CAD build for the part. Positions are in the model's coordinates, mm. Face numbers are marked on the shaded views. Give positions to 0.01 mm unless a question says otherwise; leave off trailing zeros. Loops run counter-clockwise (first coordinate to the right, second up) from the corner with the lowest first, then second, coordinate; pieces in that order, holes last. Notation, with made-up numbers: M -7,6 L 14,6 A22 cw 14,25 Z; hole C -27,29.5 d9. An arc over 180 degrees is marked long. Answer as CSV lines item,"result".
Autodesk Inventor part; units mm, degrees
ref_plane "Work Plane1" through (0, 0, 19.685) normal (0, 0, 1) x (1, 0, 0)
ref_plane "YZ Plane" through (0, 0, 0) normal (1, 0, 0) x (0, 1, 0)
ref_plane "XZ Plane" through (0, 0, 0) normal (0, 1, 0) x (-1, 0, 0)
sketch "Sketch1" plane through (0, 0, 0) normal (0, 0, 1) x (1, 0, 0)
  line L0 (0, 6.35) -> (0, 53.34)
  line L1 (0, 53.34) -> (-19.05, 53.34)
  line L2 (-19.05, 53.34) -> (-19.05, 55.245)
  line L3 (-12.7, 48.895) -> (-6.35, 48.895)
  line L4 (-6.35, 48.895) -> (-6.35, 13.335)
  line L5 (-6.35, 13.335) -> (-19.05, 13.335)
  line L6 (-19.05, 13.335) -> (-19.05, 12.7)
  line L7 (-12.7, 8.89) -> (-6.35, 8.89)
  line L8 (-6.35, 8.89) -> (-6.35, 0)
  line L9 (-6.35, 0) -> (0, 0)
  line L10 (-19.05, 55.245) -> (-19.05, 40.005)
  line L11 (-19.05, 40.005) -> (-12.7, 40.005)
  line L12 (-12.7, 40.005) -> (-12.7, 48.895)
  line L13 (-19.05, 12.7) -> (-19.05, 0)
  line L14 (-19.05, 0) -> (-12.7, 0)
  line L15 (-12.7, 0) -> (-12.7, 8.89)
  line L16 (0, 0) -> (0, 6.35)
  point P0 (-19.05, 53.34)
  point P1 (-19.05, 11.43)
  dimension "d1" = 35.56
  dimension "d2" = 4.445
  dimension "d3" = 4.445
  dimension "d4" = 6.35
  dimension "d6" = 6.35
  dimension "d7" = 6.35
  dimension "d13" = 13.335
  dimension "d14" = 13.335
extrude "Extrusion1" add sketch "Sketch1" along normal mid plane 3.81
ref_plane "Work Plane1" through (0, 0, 19.685) normal (0, 0, 1) x (1, 0, 0)
mirror "Mirror1" about plane through (0, 0, 19.685) normal (0, 0, 1) of "Extrusion1"
sketch "Sketch4" plane through (0, 0, 19.685) normal (0, 0, 1) x (1, 0, 0)
  line L0 (-6.35, 8.89) -> (-6.35, 0)
  line L1 (-6.35, 0) -> (50.8, 0)
  line L2 (50.8, 0) -> (50.8, 6.35)
  line L3 (50.8, 6.35) -> (-6.35, 6.35)
  line L4 (-6.35, 6.35) -> (-6.35, 0)
  point P0 (0, 0)
  dimension "d23" = 57.15
  dimension "d24" = 6.35
extrude "Extrusion4" add sketch "Sketch4" along normal mid plane 50.8
sketch "Sketch5" plane through (-6.35, 6.35, 45.085) normal (0, 1, 0) x (1, 0, 0)
  line L0 (0, 50.8) -> (57.15, 50.8) construction
  line L1 (6.35, 50.8) -> (6.35, -0.1726) construction
  line L2 (57.15, 50.8) -> (57.15, 0) construction
  line L3 (6.35, 50.8) -> (57.15, 0) construction
  line L4 (6.35, -0.1726) -> (57.15, 50.8) construction
  circle A0 centre (31.75, 25.3137) radius 19.05
  point P0 (6.35, 45.085)
  dimension "d27" = 38.1
extrude "Extrusion5" cut sketch "Sketch5" against normal through all
fillet "Fillet1" radius 3.175 4 edges at (-6.35, 3.175, 45.085) (50.8, 3.175, 45.085) (50.8, 3.175, -5.715) (-6.35, 3.175, -5.715)
ref_plane "Work Plane2" through (0, 0, 19.685) normal (0, 0, 1) x (1, 0, 0)
sketch "Sketch6" plane through (-19.05, 53.34, 41.275) normal (0, 0, 1) x (1, 0, 0)
  line L0 (19.05, 0) -> (19.05, -46.99)
  line L1 (66.675, -46.99) -> (15.875, -46.99)
  line L2 (19.05, -46.99) -> (19.05, 0)
  line L3 (19.05, -30.4922) -> (28.575, -46.99)
  line L4 (28.575, -46.99) -> (19.05, -46.99)
  line L5 (19.05, -46.99) -> (19.05, -30.4922)
  point P0 (19.05, -53.34)
  dimension "d37" = 9.525
  dimension "d38" = 60
extrude "Extrusion6" add sketch "Sketch6" against normal up to surface (3.81 mm away)
fillet "Fillet2" radius 3.175 2 edges at (9.525, 6.35, 39.37) (0, 22.8478, 39.37)
sketch "Sketch7" plane through (0, 0, -1.905) normal (0, 0, -1) x (-1, 0, 0)
  line L0 (0, 53.34) -> (0, 6.35)
  line L1 (3.175, 6.35) -> (-47.625, 6.35)
  line L2 (0, 6.35) -> (0, 53.34)
  line L3 (0, 22.8478) -> (0, 6.35)
  line L4 (0, 6.35) -> (-9.525, 6.35)
  line L5 (-11.3581, 6.35) -> (6.35, 6.35)
  line L6 (-9.525, 6.35) -> (0, 22.8478)
  point P0 (0, 0)
  dimension "d42" = 60
  dimension "d43" = 9.525
extrude "Extrusion7" add sketch "Sketch7" against normal up to surface (3.81 mm away)
fillet "Fillet3" radius 3.175 2 edges at (0, 22.8478, 0) (9.525, 6.35, 0)
equation "\"d11\" = width"
equation "\"d15\" = oneHalfSpacing"
equation "\"width\" = 3.81"
equation "\"spacing\" = 39.37"
equation "\"oneHalfSpacing\" = 0.5 * spacing"
properties part number "round_1_5_inchHoleV01"
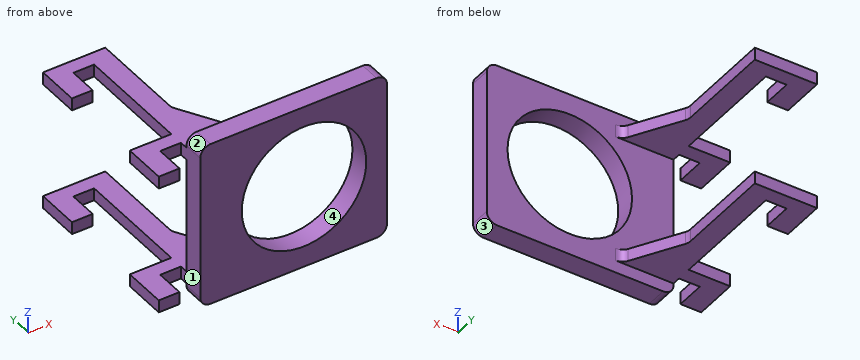
1) Band-saw the part on B-B on z = 4. Give the cut face in (x, y).
Answer below:
outline,"M -6.35,0 L 14.72,0 L 14.72,6.35 L -6.35,6.35 Z; M 36.08,0 L 50.8,0 L 50.8,6.35 L 36.08,6.35 Z"
2) Band-saw the part on C-C on x = -2. Give the cut face in (y, z) (3 decimals), and give its area (3 significant figures).
Answer below:
outline,"M 0,-5.715 L 6.35,-5.715 L 6.35,-1.905 L 53.34,-1.905 L 53.34,1.905 L 6.35,1.905 L 6.35,37.465 L 53.34,37.465 L 53.34,41.275 L 6.35,41.275 L 6.35,45.085 L 0,45.085 Z"
area,"681 mm^2"
3) Band-saw the part on D-D on x = 46. Give the cut face in (y, z) (3 decimals).
Answer below:
outline,"M 0,-5.715 L 6.35,-5.715 L 6.35,45.085 L 0,45.085 Z"
4) Mould opens along X. For the marked faces 1, 2, 3 and 4 say: +X half, -X half, draft (parallel to the pull), parting line (faces both ways), or undercut.
Answer below:
face 1,"undercut"
face 2,"-X half"
face 3,"+X half"
face 4,"undercut"
5) Drill centre lines: line 1 (Z direction, x = 25.4, y = 4.75) (3 decimals); line 2 (X direction, y = 25.5, z = 37.5); line 3 (Y direction, x = -6, z = 24). Where is each one in solid material? Low to high. Write a range as from..to.
Answer below:
line 1,"z = -5.715..0.721, 38.821..45.085"
line 2,"x = -6.35..0"
line 3,"y = 0..6.35"
6) Flat gauge pins, fed straight in: pin 1 (1.1 mm diameter, centred on y = 31.5, z = -0.5, fed in from +X); pin 2 (8 mm diameter, centred on x = 38.5, z = 14, fed in from +Y); pin 3 (6 mm diameter, centred on x = 32, z = 3, fed in from +Y); pin 4 (4 mm diameter, centred on x = -10, z = 39.5, fed in from -Y). Where does each tip first touch, or does it go through?
Answer below:
pin 1,"stops at x = 0"
pin 2,"passes through"
pin 3,"stops at y = 6.35"
pin 4,"stops at y = 8.89"
7) Band-saw the part on A-A on x = 25.4. Give the cut face in (y, z) (3 decimals), and give its area (3 significant figures).
Answer below:
outline,"M 0,-5.715 L 6.35,-5.715 L 6.35,0.721 L 0,0.721 Z; M 0,38.821 L 6.35,38.821 L 6.35,45.085 L 0,45.085 Z"
area,"80.6 mm^2"
